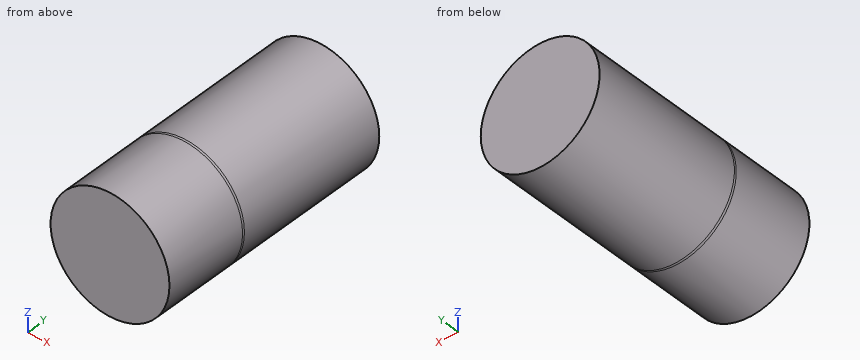
from build123d import *

# Parameters (mm, degrees)
F1_R     = 13.608601514
F2_DEPTH = 36.068
F4_DEPTH = 36.576
F5_DEPTH = 56.134


# Not quite as in the source:
# - the program builds the solid bodies; features that only make, move or delete a surface that nothing else refers to are left out


with BuildPart() as f2:
    # F1 (on Front) → F2 (new body)
    with BuildSketch(Plane.XZ):
        Circle(F1_R)
    extrude(amount=-F2_DEPTH)

    # F4 (add): a face of the model
    f4_faces = [f2.faces().sort_by_distance(p)[0] for p in [
        (0, 36.068, 0),
    ]]
    extrude(f4_faces, amount=-F4_DEPTH)

    # F5 (add): a face of the model
    f5_faces = [f2.faces().sort_by_distance(p)[0] for p in [
        (0, 36.068, 0),
    ]]
    extrude(f5_faces, amount=-F5_DEPTH)


solid = f2.part
The listing builds one solid part. Answer for the finished solid, in the listing's coordinates (mm). Round coordinates to 2 decimals unless told otherwise and drop trailing zeros. Order: outer loops, then holes, each group sorted by start corner. A loop starts at its lowest first (then second) coordinate and runs counter-clockwise, first axis right, second up. Notation, with made-up numbers: (25.25, -26) -> (80.25, -26) arc R6 cw to (80.25, -17) -> close; hole circle Ø5 at (29.25, -30). An arc over 180 degrees is marked (long way). Write each question's results on one line, items separated by ' | '. Start each with the question number.
Q1. Find section A-A (y = -12). Determine the outline of the cut face in (x, z).
Q2. Straight lines are drawn through the part: probe 1 along X at (y, z) = (-10, -0.25); probe 2 along X at (y, z) = (-6.5, 9). For each, find the intervals that lie inside material, in ascending order. Write a range as from..to.
Q3. Find section C-C (x = 10). Determine the outline of the cut face in (y, z), then the cut area to 3 significant figures.
Q4. Find section B-B (x = -4.25). Determine the outline of the cut face in (y, z).
Q5. Each of these flat-tipped pins is pushed along its axis until it touches: pin 1 (2 mm diameter, centred on x = -5, y = -3.5, fed in from -Z); pin 2 (2 mm diameter, centred on x = 2, y = 29.5, fed in from -Z); pin 3 (2 mm diameter, centred on x = -2, y = 7.5, fed in from +Z). Where does it stop, or does it pass through?
Worked answers:
1) outline: circle Ø27.22 at (0, 0)
2) probe 1: x = -13.61..13.61 | probe 2: x = -10.21..10.21
3) outline: (-20.07, -9.23) -> (36.07, -9.23) -> (36.07, 9.23) -> (-20.07, 9.23) -> close | area: 1,040 mm2
4) outline: (-20.07, -12.93) -> (36.07, -12.93) -> (36.07, 12.93) -> (-20.07, 12.93) -> close
5) pin 1: stops at z = -13.01 | pin 2: stops at z = -13.57 | pin 3: stops at z = 13.57
